For this review, use the dimensioned drawing (mm, ordinates from the lowest corner) and the shaded views. A direction names the side the tool comes from. Coordinates: 2 decimals unless noted, no trailing zeros. Write each loop counter-clockwise with the first axis right and the second up, starting at its lowest first coordinate (ties: lowest second). Pieces come first, ordered by that corner, then holes. Notation, with made-up numbers: M -15.5,-36.75 L -3.5,-36.75 A9 ccw -3.5,-32.75 Z; hole C 84.5,63 d3. An arc over 180 degrees is marked long. Return JSON: item names as keys, results as strings.
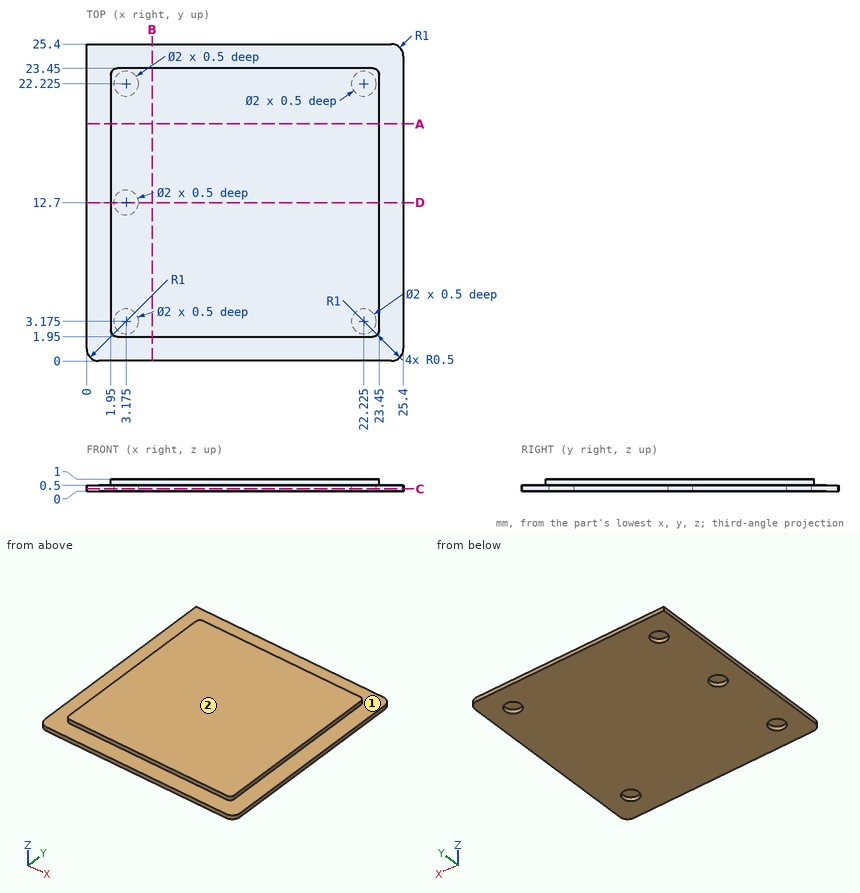
1. For the marked faces 1 and 2, list the 3-axis set-ups (+Z, -Z, +X, -X, +Y, -Y) from which the entire face can be reached by the end or side of a thin tool; tool diameter is ignored.
Checks:
{"face 1": "+Z", "face 2": "+Z, +X, -X, +Y, -Y"}
2. We need section A-A (y = 19). State the section outline as (x, z) points, plus the area to 4 significant figures.
Checks:
{"outline": "M 0,0 L 25.4,0 L 25.4,0.5 L 23.45,0.5 L 23.45,1 L 1.95,1 L 1.95,0.5 L 0,0.5 Z", "area": "23.45 mm2"}
3. We need section D-D (y = 12.7). State the section outline as (x, z) points (3 decimals), plus the area to 4 significant figures.
Checks:
{"outline": "M 0,0 L 2.175,0 L 2.175,0.5 L 4.175,0.5 L 4.175,0 L 25.4,0 L 25.4,0.5 L 23.45,0.5 L 23.45,1 L 1.95,1 L 1.95,0.5 L 0,0.5 Z", "area": "22.45 mm2"}
4. We need section C-C (z = 0.2). State the section outline as (x, y) points (3 decimals), plus the area to 3 significant figures.
Checks:
{"outline": "M 0,1 A1 ccw 1,0 L 24.4,0 A1 ccw 25.4,1 L 25.4,24.4 A1 ccw 24.4,25.4 L 0,25.4 Z; hole C 3.175,3.175 d2; hole C 3.175,12.7 d2; hole C 3.175,22.225 d2; hole C 22.225,3.175 d2; hole C 22.225,22.225 d2", "area": "629 mm2"}
5. Clearance check with a flat-ended pin moving along its axis: pin 1 Ø0.6 at (x, y) = (22.5, 3.5) entering from -Z. State where the tip first meets the part, or that it passes through.
Checks:
{"pin 1": "z = 0.5"}
6. Wall thickness on L1, parallel to X at y = 21.5, z = 0.2; L2, parallel to X at y = 12.75, z = 0.25; L3, parallel to Y at x = 10.5, z = 0.7: over which ranges is each line inside the solid? List them lowest first. Write a range as from..to.
Checks:
{"L1": "0..2.49, 3.86..21.54, 22.91..25.4", "L2": "0..2.18, 4.17..25.4", "L3": "1.95..23.45"}
